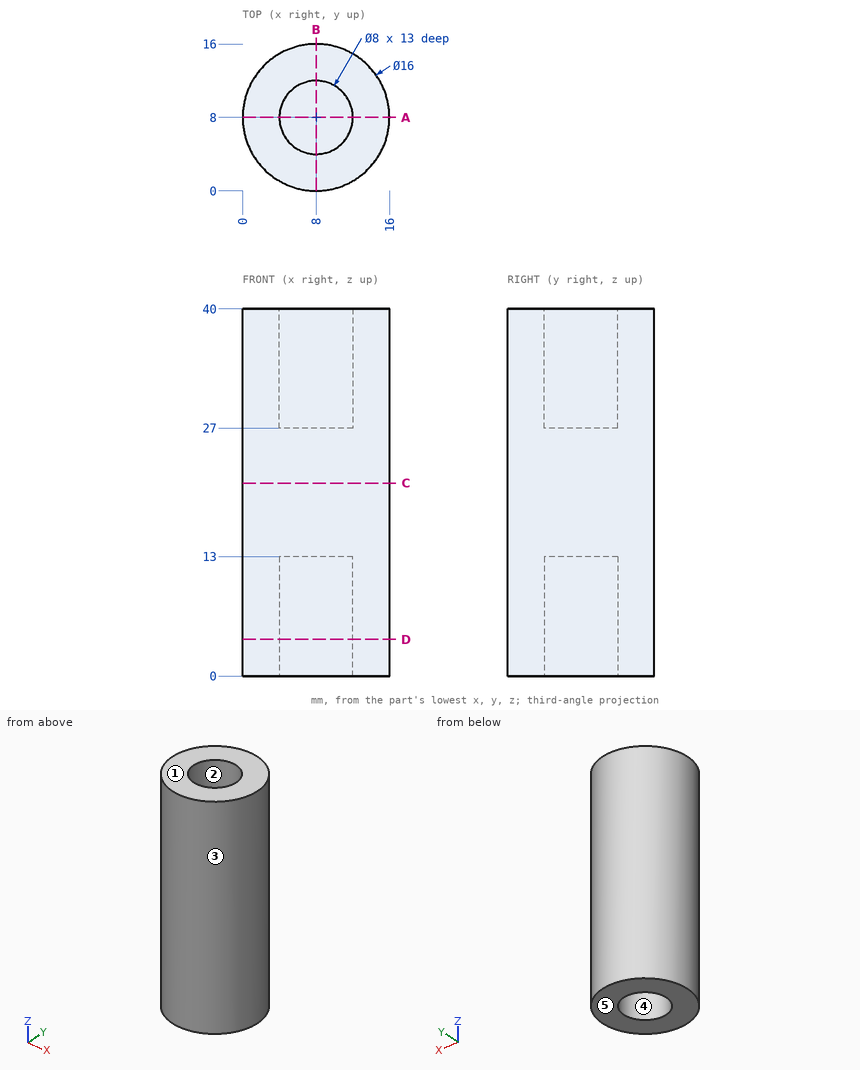
Study the drawing (mm; zero at the part's minimum x, y, z) and answer. A direction names the side the tool comes from. Give positions to 0.01 mm unless a question says otherwise; leave off trailing zeros. Order: outer loops, then holes, each group sorted by start corner. A loop starts at its lowest first (then second) coordinate and runs counter-clockwise, first axis right, second up. Notation, with made-up numbers: (79.25, 83.25) -> (106.25, 83.25) arc R26 cw to (106.25, 109.25) -> close; hole circle Ø10 at (45.5, 80.5). An arc over 180 degrees is marked (long way). Write item = value, one per line.
1. A cutting plane is placed at A-A, the plane y = 8. Write down the section's boundary in (x, z).
Numbers:
outline = (0, 0) -> (4, 0) -> (4, 13) -> (12, 13) -> (12, 0) -> (16, 0) -> (16, 40) -> (12, 40) -> (12, 27) -> (4, 27) -> (4, 40) -> (0, 40) -> close
2. The mould has two halves that part along Y. Classify the marked faces 3, 4 and 5: +Y half, -Y half, draft (parallel to the pull), parting line (faces both ways), or undercut.
Numbers:
face_3 = parting line
face_4 = undercut
face_5 = draft
3. Given pin 1 (6.5 mm diameter, centred on x = 9.5, y = 7.5, fed in from -Z); pin 2 (3 mm diameter, centred on y = 4.5, z = 17, fed in from +X); pin 3 (3 mm diameter, centred on y = 5, z = 7.5, fed in from +X); pin 4 (2 mm diameter, centred on y = 5, z = 8.5, fed in from -X), each flat-ended and moving along its own axis, determine where each tip first touches the part or whether it passes through.
Numbers:
pin_1 = 0
pin_2 = 15.75
pin_3 = 15.86
pin_4 = 0.25
4. A cutting plane is placed at D-D, the plane z = 4. Write down the section's boundary in (x, y).
Numbers:
outline = circle Ø16 at (8, 8); hole circle Ø8 at (8, 8)
5. A cutting plane is placed at C-C, the plane z = 21. Write down the section's boundary in (x, y).
Numbers:
outline = circle Ø16 at (8, 8)
6. Straight lines are drawn through the part: line 1 along Y through (x, z) = (8, 7.25); line 2 along Z through (x, y) = (10.25, 8.5); line 3 along Y through (x, z) = (9, 32.5). For each, find the intervals that lie inside material, in ascending order.
Numbers:
line_1 = 0 to 4, 12 to 16
line_2 = 13 to 27
line_3 = 0.06 to 4.13, 11.87 to 15.94
7. For the marked faces 1 and 2, determine the directions among +Z, -Z, +X, -X, +Y, -Y from which every point of the face is accessible in a straight line to the end or side of a thin tool.
Numbers:
face_1 = +Z, +X, -X, +Y, -Y
face_2 = +Z
